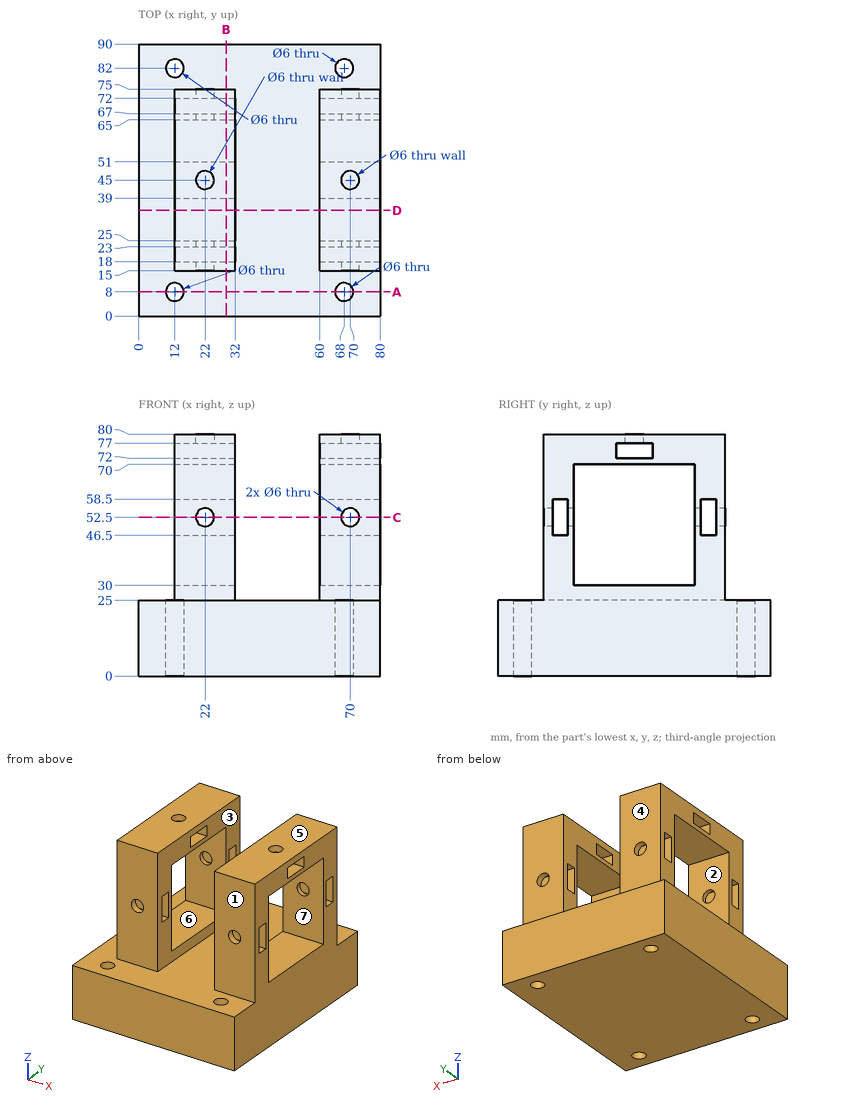
Source: three-view drawing plus pictorial views. Frame: mm from the lowest corner of the part. A direction names the side the tool comes from. Coordinates: 2 decimals unless noted, no trailing zeros. Order: outer loops, then holes, each group sorted by start corner. A loop starts at its lowest first (then second) coordinate and runs counter-clockwise, first axis right, second up. Notation, with made-up numbers: M -6.75,62.25 L 26.25,62.25 A15 ccw 26.25,85.25 Z; hole C -37.75,-36.5 d1. An arc over 180 degrees is marked long. Write each question's results on one line, items separated by ' | '. Start each with the question number.
1. Section A-A, the plane y = 8. Return the cut outline in (x, z), then the cut area to 3 significant figures.
2. Section B-B, the plane x = 29. Return the cut outline in (y, z).
3. Section C-C, the plane z = 52.5. State how many separate pieces and enclosed holes the cut face has, then the cut area to 3 significant figures.
4. Draft query along Z for the marked faces 4, 5, 6 and 7. Return one class per face: +Z half, -Z half, draft (parallel to the pull), parting line (faces both ways), or undercut.
5. Reachability of the marked faces 1, 2 and 3 from +Z, -Z, +X, -X, +Y, -Y: full face, straight path, thin tool, end or side. Return the list, or none.
6. Pin query (flat end, axial travel): pin 1 (4 mm diameter, centred on x = 16.5, z = 68.5, fed in from -Y); pin 2 (16.5 mm diameter, centred on y = 48, z = 39.5, fed in from -X); pin 3 (22 mm diameter, centred on x = 20, z = 40, fed in from +Y). Return the tip coordinate at first contact, or that it passes through.
7. Section D-D, the plane y = 35. Return the cut outline in (x, z).
8. Material intervals for L1, parallel to Y at x = 12, z = 9.25; L2, parallel to Z at x = 70, y = 73.5; L3, parallel to X at y = 16, z = 52, sorted ascending.
Solution:
1) outline: M 0,0 L 9,0 L 9,25 L 0,25 Z; M 15,0 L 65,0 L 65,25 L 15,25 Z; M 71,0 L 80,0 L 80,25 L 71,25 Z | area: 1,700 mm²
2) outline: M 0,0 L 90,0 L 90,25 L 75,25 L 75,80 L 15,80 L 15,25 L 0,25 Z; hole M 18,46.5 L 23,46.5 L 23,58.5 L 18,58.5 Z; hole M 25,30 L 65,30 L 65,70 L 25,70 Z; hole M 39,72 L 51,72 L 51,77 L 39,77 Z; hole M 67,46.5 L 72,46.5 L 72,58.5 L 67,58.5 Z
3) separate pieces: 16 | enclosed holes: 0 | area: 280 mm²
4) face 4: draft | face 5: +Z half | face 6: undercut | face 7: undercut
5) face 1: +Z, +X, -X, -Y | face 2: +X, -X | face 3: +Z, +Y, -Y
6) pin 1: y = 15 | pin 2: through | pin 3: y = 75
7) outline: M 0,0 L 80,0 L 80,30 L 60,30 L 60,25 L 32,25 L 32,30 L 12,30 L 12,25 L 0,25 Z; M 12,70 L 32,70 L 32,80 L 12,80 Z; M 60,70 L 80,70 L 80,80 L 60,80 Z
8) L1: 0 to 5, 11 to 79, 85 to 90 | L2: 0 to 49.5, 55.5 to 80 | L3: 12 to 19.04, 24.96 to 32, 60 to 67.04, 72.96 to 80
